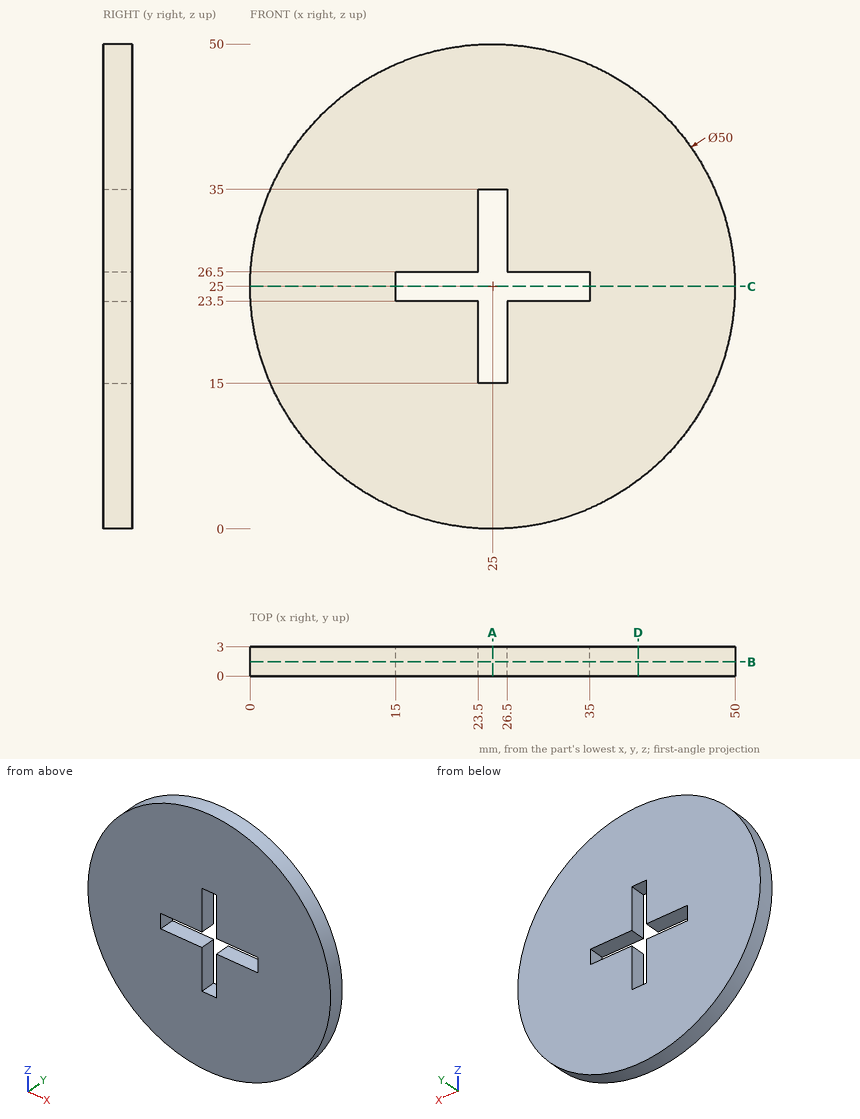
Study the drawing (mm; zero at the part's minimum x, y, z) and answer. Give positions to 0.01 mm unless a question says otherwise; leave off trailing zeros. Loops run counter-clockwise (first coordinate to the right, second up) from the corner with the lowest first, then second, coordinate; pieces in that order, holes last. Notation, with made-up numbers: M -7.5,58.5 L -3.5,58.5 A18 cw -3.5,90.5 Z; hole C 53.25,-35 d5. An arc over 180 degrees is marked long. Use CSV: the item, a comma, the result in double quotes.
1) Consider L1, parallel to X at y = 0.5, z = 25.5 (3 decimals); L2, parallel to Z at x = 21.5, y = 0.15; L3, parallel to Z at x = 33.5, y = 0.25. Determine where each line is inside the solid, lowest interval first.
Answer:
L1,"0.005 to 15, 35 to 49.995"
L2,"0.25 to 23.5, 26.5 to 49.75"
L3,"1.49 to 23.5, 26.5 to 48.51"
2) Find section C-C on z = 25. Write down the section's boundary in (x, y).
Answer:
outline,"M 0,0 L 15,0 L 15,3 L 0,3 Z; M 35,0 L 50,0 L 50,3 L 35,3 Z"
3) Find section B-B on y = 1.45. Write down the section's boundary in (x, z).
Answer:
outline,"C 25,25 d50; hole M 15,23.5 L 23.5,23.5 L 23.5,15 L 26.5,15 L 26.5,23.5 L 35,23.5 L 35,26.5 L 26.5,26.5 L 26.5,35 L 23.5,35 L 23.5,26.5 L 15,26.5 Z"
4) Find section A-A on x = 25. Write down the section's boundary in (y, z), plus the area to 3 significant figures.
Answer:
outline,"M 0,0 L 3,0 L 3,15 L 0,15 Z; M 0,35 L 3,35 L 3,50 L 0,50 Z"
area,"90.0 mm^2"
5) Given P1, Ø0.9, axis at y = 1, z = 18, coming from the +X side; P2, Ø1.5, axis at x = 29.5, y = 1, coming from the +Z side; P3, Ø1.5, axis at x = 24.5, y = 1, coming from the -Z side, each flat-ended and moving along its own axis, determine where each tip first touches the part or whether it passes through.
Answer:
P1,"x = 49.13"
P2,"z = 49.72"
P3,"z = 0"
6) Find section D-D on x = 40. Write down the section's boundary in (y, z), plus the area to 3 significant figures.
Answer:
outline,"M 0,5 L 3,5 L 3,45 L 0,45 Z"
area,"120 mm^2"
